Autodesk Inventor part; units mm, degrees
ref_plane "YZ Plane" through (0, 0, 0) normal (1, 0, 0) x (0, 1, 0)
ref_plane "XZ Plane" through (0, 0, 0) normal (0, 1, 0) x (-1, 0, 0)
ref_plane "XY Plane" through (0, 0, 0) normal (0, 0, 1) x (1, 0, 0)
sketch "Sketch3" plane through (0, 0, 0) normal (1, 0, 0) x (0, 1, 0)
  line L0 (0, 0) -> (0, -35)
  line L1 (-17.5736, -77.4264) -> (-42.3223, -102.1751)
  arc A0 (-17.5736, -77.4264) -> (0, -35) centre (-60, -35) ccw
  point P0 (0, -59.8528)
  point P1 (0, -15)
  point P2 (-31.7157, -91.5685)
  dimension "d34" = 59.8528
  dimension "d36" = 135
  dimension "d37" = 60
  dimension "d40" = 15
  dimension "d41" = 15
  dimension "d50" = 35
sketch "Sketch1" plane through (0, 0, 0) normal (0, 0, 1) x (1, 0, 0)
  circle A0 centre (0, 0) radius 17.5
  circle A1 centre (0, 0) radius 21
  dimension "d1" = 42
  dimension "d2" = 35
sweep "Sweep1" add profiles "Sketch1" path "Sketch3"
hole "Hole3" at (0, 0, -15) at (0, -31.7157, -91.5685) direction (-1, 0, 0) diameter 6.647 end through all
fillet "Fillet3" radius 2 2 edges at (-21, 0, 0) (-21, -42.3223, -102.1751)
properties part number "55-6" material "Iron, Cast"
Geometry: final body of the model. Coordinates: model frame, mm. A direction names the side the tool comes from. Give positions to 0.01 mm unless a question says otherwise; leave off trailing zeros. Write each loop counter-clockwise with the first axis right and the second up, starting at its lowest first coordinate (ties: lowest second). Pieces come first, ordered by that corner, then holes. Notation, with made-up numbers: (-39, 78.25) - (8, 78.25) arc R14 ccw to (8, 86.25) - close; hole circle Ø3 at (1, 11). An arc over 180 degrees is marked (long way). Return JSON: item names as keys, results as strings. Group by question number.
1) Set-up query: faces 5 (the cylindrical face through (16.69, -5.26, -17.74)), 6 (the cylindrical face through (-19.12, -31.86, -88.25)). Return all of +Z, -Z, +X, -X, +Y, -Y with unobstructed straight access to the full face (end or side cutting, diameter ignored); none if empty.
2) First-contact query: P1, Ø6, axis at x = 8, z = -78.5, coming from the +Y side; P2, Ø3, axis at y = -37.5, z = -70.5, coming from the -X side; P3, Ø5, axis at y = -23.5, z = -95, coming from the +X side. Flat tips, straight axial feed; report the tip coordinate or a pass-through.
3) Line query: line 1 (X direction, y = -35.5, z = -94); line 2 (Y direction, x = 0, z = -15); line 3 (X direction, y = 14.5, z = -32). Output: solid intervals per line, ascending.
4) Mould query, pull axis Y, two halves, no side actions, for faces 1 (the flat face through (-17, -45.8, -98.7)), 2 (the cylindrical face through (-19.12, -0.15, -11.68)), 3 (the flat face through (6, -17, 0)), 4 (the cylindrical face through (20.03, -6.31, -18.73)). Classes: released by +Y, released by -Y, zero draft, split by the parting line, or undercut.
5) Section A-A on z = -15. Return the cut outline in (x, y).
Filled in:
{
 "1": {"face 5": "+Z", "face 6": "-X"},
 "2": {"P1": "stops at y = 8.72", "P2": "stops at x = -11.63", "P3": "stops at x = 20.2"},
 "3": {"line 1": "x = -20.98 to -17.47, 17.47 to 20.98", "line 2": "y = -21 to -17.5, 17.5 to 21", "line 3": "x = -15.19 to -9.8, 9.8 to 15.19"},
 "4": {"face 1": "released by -Y", "face 2": "undercut", "face 3": "zero draft", "face 4": "split by the parting line"},
 "5": {"outline": "(-20.74, -3.32) arc R21 ccw (long way) to (-20.74, 3.32) - (-17.18, 3.32) arc R17.5 cw (long way) to (-17.18, -3.32) - close"}
}
